Geometry: final body of the model. Coordinates: model frame, mm. A direction names the side the tool comes from. Coordinates: 2 decimals unless noted, no trailing zeros. Write each loop counter-clockwise with the first axis right and the second up, starting at its lowest first coordinate (ties: lowest second). Pieces come first, ordered by that corner, then holes. Notation, with made-up numbers: (-21.5, 79) -> (5.5, 79) arc R24 cw to (5.5, 110) -> close; hole circle Ø11 at (75, 56). An arc over 180 degrees is marked (long way). One line per item, written item: value. Start each with the question number.
from build123d import *

# Parameters (mm, degrees)
POCKET_DEPTH = 13.001
CHAMFER_SIZE = 0.5


with BuildPart() as part:
    # Sketch → Revolution (revolve)
    with BuildSketch(Plane.YZ):
        Polygon((11.2, 17), (0, 17), (0, 0), (13, 0), (13, 3.9), (11.2, 3.9), align=None)
    revolve(axis=Axis((0, 0, 0), (0, 1, 0)))

    # Sketch001 → Pocket (cut, through all)
    with BuildSketch(Plane.XZ):
        with BuildLine():
            ThreePointArc((1.1, 1.161895), (-1.6, 0), (1.1, -1.161895))
            Line((1.1, 1.161895), (1.1, -1.161895))
        make_face()
    extrude(amount=-POCKET_DEPTH, mode=Mode.SUBTRACT)

    # Chamfer
    chamfer_edges = [part.edges().sort_by_distance(p)[0] for p in [
        (0, 0, -17),
        (1.1, 0, 0),
        (-1.6, 0, 0),
    ]]
    chamfer(chamfer_edges, length=CHAMFER_SIZE)


solid = part.part
Q1. Cut plane B-B on x = 0. Output: boundary loops of the cut face in (y, z), and give its area (3 significant figures).
Q2. Draft query along X for faces 1 (the flat face through (-3, 0, 0)), 2 (the conical face through (-1.734, 0.365, 0.059)), 3 (the cylindrical face through (2.64, 12.09, -2.87)). Return one class per face: pulls with the +X half, pulls with the -X half, needs draft (parallel to the pull), parting line crosses it, or undercut.
Q3. Line query: L1, parallel to Y at x = -8, z = 1.5; L2, parallel to X at y = 9.5, z = 14; L3, parallel to X at y = 7.75, z = 6.5. Output: solid intervals per line, ascending. Write a range as from..to.
Q4. Cut plane D-D on y = 12. Output: boundary loops of the cut face in (x, z).
Q5. Cut plane A-A on z = 0. Output: boundary loops of the cut face in (x, y), and give its area (3 significant figures).
Q6. Cut plane C-C on y = 1.5. Output: boundary loops of the cut face in (x, z).
Q7. Access query for faces 4 (the flat face through (1.1, 7, 0)), 5 (the flat face through (0, 13, -2)). Directions: +Z, -Z, +X, -X, +Y, -Y. A direction counts if a zero-diameter tool reaches every point of the face in a straight line with its end or side. Return the directions, or none.
Q8. First-contact query: P1, Ø4, axis at y = 7, z = -4.5, coming from the -X side; P2, Ø2, axis at x = -11, z = -6.5, coming from the +Y side; P3, Ø5, axis at x = 12.5, y = 8.5, coming from the -Z side. Flat tips, straight axial feed; report the tip coordinate or a pass-through.
Solution:
1. outline: (0, -16.5) -> (0.5, -17) -> (11.2, -17) -> (11.2, -3.9) -> (13, -3.9) -> (13, -1.6) -> (0.5, -1.6) -> (0, -2.1) -> close; (0, 2.1) -> (0.5, 1.6) -> (13, 1.6) -> (13, 3.9) -> (11.2, 3.9) -> (11.2, 17) -> (0.5, 17) -> (0, 16.5) -> close
1. area: 353 mm²
2. face 1: needs draft
2. face 2: undercut
2. face 3: parting line crosses it
3. L1: 0..11.2
3. L2: -9.64..9.64
3. L3: -15.71..15.71
4. outline: circle Ø7.8 at (0, 0); hole (1.1, -1.16) -> (1.1, 1.16) arc R1.6 ccw (long way) to start
5. outline: (-17, 0.5) -> (-16.5, 0) -> (-2.1, 0) -> (-1.6, 0.5) -> (-1.6, 13) -> (-3.9, 13) -> (-3.9, 11.2) -> (-17, 11.2) -> close; (1.1, 0.5) -> (1.6, 0) -> (16.5, 0) -> (17, 0.5) -> (17, 11.2) -> (3.9, 11.2) -> (3.9, 13) -> (1.1, 13) -> close
5. area: 359 mm²
6. outline: circle Ø34 at (0, 0); hole (1.1, -1.16) -> (1.1, 1.16) arc R1.6 ccw (long way) to start
7. face 4: +Y, -Y
7. face 5: +Z, -Z, +X, -X, +Y
8. P1: x = -16.82
8. P2: y = 11.2
8. P3: z = -13.75
